from build123d import *

# Parameters (mm, degrees)
F0_W          = 30
F0_H          = 10
F1_DEPTH      = 30
F2_R          = 2.3
F3_DEPTH      = 30.001
F4_W          = 20
F4_H          = 50
F5_DEPTH      = 13
F5_DEPTH_BACK = 15.001


with BuildPart() as f1:
    # F0 (on Front) → F1 (new body)
    with BuildSketch(Plane.XZ):
        with Locations((0, 18.2561938465)):
            Rectangle(F0_W, F0_H)
        Polygon((15, 13.2561938465), (-15, 13.2561938465), (-15, -49.2438061535), align=None)
    extrude(amount=F1_DEPTH)

    # F2 (on face) → F3 (cut, through all)
    with BuildSketch(Plane(origin=(-15, 0, 0), x_dir=(0, -1, 0), z_dir=(-1, 0, 0))):
        with Locations((15, 0)):
            Circle(F2_R)
        with Locations((15, -32.5)):
            Circle(F2_R)
    extrude(amount=-F3_DEPTH, mode=Mode.SUBTRACT)

    # F4 (on Right) → F5 (cut, two sides)
    with BuildSketch(Plane.YZ) as f5_sk:
        with Locations((-15.0000003725, -17.2735065222)):
            Rectangle(F4_W, F4_H)
    extrude(amount=-F5_DEPTH, mode=Mode.SUBTRACT)
    extrude(f5_sk.sketch, amount=F5_DEPTH_BACK, mode=Mode.SUBTRACT)


solid = f1.part
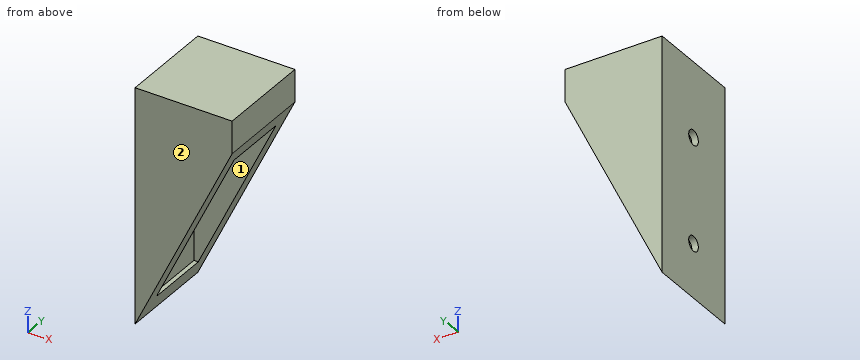
The model under review builds one solid part; all positions refer to its coordinate system, in mm. Face numbers are marked on the shaded views. A direction names the side the tool comes from. Round coordinates to 2 decimals unless told otherwise and drop trailing zeros. Write each loop counter-clockwise with the first axis right and the second up, starting at its lowest first coordinate (ties: lowest second). Pieces come first, ordered by that corner, then holes. Notation, with made-up numbers: M 19.5,15 L 46.5,15 A34 ccw 46.5,48 Z; hole C 38,24 d11. An arc over 180 degrees is marked long. Use a Markdown table: item, result. Add a question column.
Q1. To check wall thickness, follow line 1 (Y direction, x = -1, z = -7.5); line 2 (Z direction, x = -13.6, y = -15); line 3 (Z direction, x = -14.5, y = -15). State the ranges of each line that lie inside material, in increasing order.
Q2. We need section C-C, the plane y = -15. State the section outline as (x, z) points, plus the area to 3 significant figures.
Q3. We need section D-D, the plane z = -15.5. State the section outline as (x, y) points.
Q4. Machinability: for the marked faces 1 and 2, which of the approach directions +Z, -Z, +X, -X, +Y, -Y give a long, thin tool a straight path to every point of the face, cutting with its end or side? Answer none if there is none.
Q5. We need section A-A, the plane y = -9. State the section outline as (x, z) points, plus the area to 3 significant figures.
Q6. Insertion check: pin 1 (3.5 mm diameter, centred on y = -15, z = -32.5, fed in from +X); pin 2 (1 mm diameter, centred on y = -20.5, z = -20.5, fed in from +X); pin 3 (3 mm diameter, centred on x = 2.5, y = -11, fed in from -Z). Each pin has a flat end and moves straight along its axis. Give the tip position at first contact, or say it passes through.
Q7. We need section B-B, the plane z = 0. State the section outline as (x, y) points.
Findings below:
| question | item | result |
|---|---|---|
| 1 | line 1 | y = -30 to -25, -5 to 0 |
| 1 | line 2 | z = -46.33 to -34.8, -30.2 to -2.3, 2.3 to 23.26 |
| 1 | line 3 | z = -48.2 to -34.8, -30.2 to -2.3, 2.3 to 23.26 |
| 2 | outline | M -15,-49.24 L -11.65,-42.27 L -13,-42.27 L -13,-34.8 L -15,-34.8 Z; M -15,-30.2 L -13,-30.2 L -13,-2.3 L -15,-2.3 Z; M -15,2.3 L -13,2.3 L -13,7.73 L 12.35,7.73 L 15,13.26 L 15,23.26 L -15,23.26 Z |
| 2 | area | 552 mm² |
| 3 | outline | M -15,-30 L 1.2,-30 L 1.2,-25 L -13,-25 L -13,-5 L 1.2,-5 L 1.2,0 L -15,0 Z |
| 4 | face 1 | +X |
| 4 | face 2 | +Z, -Z, +X, -X, -Y |
| 5 | outline | M -15,-49.24 L -11.65,-42.27 L -13,-42.27 L -13,7.73 L 12.35,7.73 L 15,13.26 L 15,23.26 L -15,23.26 Z |
| 5 | area | 570 mm² |
| 6 | pin 1 | passes through |
| 6 | pin 2 | stops at x = -13 |
| 6 | pin 3 | stops at z = 7.73 |
| 7 | outline | M -15,-30 L 8.64,-30 L 8.64,-25 L -13,-25 L -13,-17.3 L -15,-17.3 Z; M -15,-12.7 L -13,-12.7 L -13,-5 L 8.64,-5 L 8.64,0 L -15,0 Z |
